The drawing under review shows one solid part. Ordinate dimensions are in mm from its lowest x, y, z. A direction names the side the tool comes from. Round coordinates to 2 decimals unless told otherwise and drop trailing zeros. Write each loop counter-clockwise with the first axis right and the second up, starting at its lowest first coordinate (ties: lowest second). Pieces come first, ordered by that corner, then holes. Notation, with made-up numbers: (7, 75) -> (24, 75) arc R15 cw to (24, 85) -> close; hole circle Ø8 at (31, -27). An arc over 180 degrees is marked (long way). Answer in a Markdown table with one row per item. Add a question column.
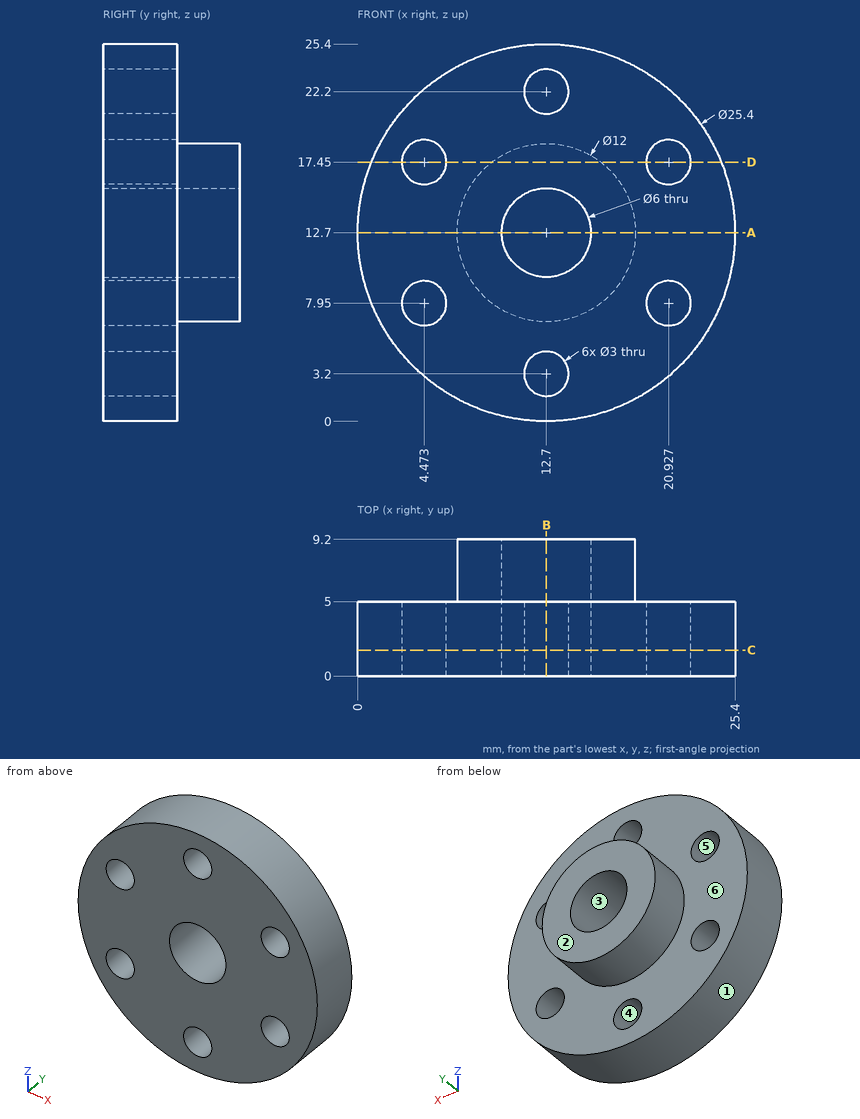
1. Add section A-A on z = 12.7. Write out the cut boundary in (x, y), plus the area to 3 significant figures.
2. Add section B-B on x = 12.7. Write out the cut boundary in (y, z).
3. Insertion check: pin 1 Ø3 at (y, z) = (7.5, 6.5) entering from +X; pin 2 Ø1 at (x, y) = (10, 2) entering from +Z; pin 3 Ø3.5 at (x, z) = (20.93, 17.45) entering from +Y. Each pin has a flat end and moves straight along its axis. Give the tip position at first contact, or say it passes through.
4. Tool access review of the marked faces 5 and 6: name each direction out of +Z, -Z, +X, -X, +Y, -Y from which nothing blocks a thin tool from reaching the whole face with its end or side.
5. Add section D-D on z = 17.45. Write out the cut boundary in (x, y), plus the area to 3 significant figures.
6. For L1, parallel to Z at x = 12.7, y = 2.2; L2, parallel to Z at x = 19.75, y = 2; L3, parallel to X at y = 0.75, z = 17.75, list the stretches that pass through material, from the lowest coordinate up.
7. Add section C-C on y = 1.75. Write out the cut boundary in (x, z), plus the area to 3 significant figures.
8. Mouldability with a two-part tool opening along Z and no side actions: class the marked faces 1, 2, 3 and 4 as pulls with the +Z half, pulls with the -Z half, needs draft (parallel to the pull), parting line crosses it, or undercut.
Filled in:
| question | item | result |
|---|---|---|
| 1 | outline | (0, 0) -> (9.7, 0) -> (9.7, 9.2) -> (6.7, 9.2) -> (6.7, 5) -> (0, 5) -> close; (15.7, 0) -> (25.4, 0) -> (25.4, 5) -> (18.7, 5) -> (18.7, 9.2) -> (15.7, 9.2) -> close |
| 1 | area | 122 mm² |
| 2 | outline | (0, 0) -> (5, 0) -> (5, 1.7) -> (0, 1.7) -> close; (0, 4.7) -> (5, 4.7) -> (5, 6.7) -> (9.2, 6.7) -> (9.2, 9.7) -> (0, 9.7) -> close; (0, 15.7) -> (9.2, 15.7) -> (9.2, 18.7) -> (5, 18.7) -> (5, 20.7) -> (0, 20.7) -> close; (0, 23.7) -> (5, 23.7) -> (5, 25.4) -> (0, 25.4) -> close |
| 3 | pin 1 | x = 16.43 |
| 3 | pin 2 | z = 25.21 |
| 3 | pin 3 | y = 5 |
| 4 | face 5 | +Y, -Y |
| 4 | face 6 | +Y |
| 5 | outline | (0.92, 0) -> (2.97, 0) -> (2.97, 5) -> (0.92, 5) -> close; (5.97, 0) -> (19.43, 0) -> (19.43, 5) -> (16.37, 5) -> (16.37, 9.2) -> (9.03, 9.2) -> (9.03, 5) -> (5.97, 5) -> close; (22.43, 0) -> (24.48, 0) -> (24.48, 5) -> (22.43, 5) -> close |
| 5 | area | 119 mm² |
| 6 | L1 | 0 to 1.7, 4.7 to 9.7, 15.7 to 20.7, 23.7 to 25.4 |
| 6 | L2 | 2.14 to 7.02, 8.88 to 16.52, 18.38 to 23.26 |
| 6 | L3 | 1.05 to 3, 5.94 to 19.46, 22.4 to 24.35 |
| 7 | outline | circle Ø25.4 at (12.7, 12.7); hole circle Ø3 at (4.47, 7.95); hole circle Ø3 at (4.47, 17.45); hole circle Ø6 at (12.7, 12.7); hole circle Ø3 at (12.7, 3.2); hole circle Ø3 at (12.7, 22.2); hole circle Ø3 at (20.93, 7.95); hole circle Ø3 at (20.93, 17.45) |
| 7 | area | 436 mm² |
| 8 | face 1 | parting line crosses it |
| 8 | face 2 | needs draft |
| 8 | face 3 | undercut |
| 8 | face 4 | undercut |
